Could you check a few things on this model? Use its own coordinates, in mm. A direction names the side the tool comes from. Round coordinates to 2 decimals unless told otherwise and drop trailing zeros. Loops run counter-clockwise (first coordinate to the right, second up) from the corner with the lowest first, then second, coordinate; pieces in that order, holes last.
from build123d import *

# Parameters (mm, degrees)
FILLET1_R          = 2
CHAMFER1_SIZE      = 1.5
CUT_EXTRUDE1_DEPTH = 2
CIRPATTERN1_COUNT  = 8
CUT_EXTRUDE2_DEPTH = 2
CIRPATTERN2_COUNT  = 6


with BuildPart() as part:
    # Sketch2 → Revolve1 (revolve)
    with BuildSketch(Plane(origin=(0, 0, 0), x_dir=(0, 0, -1), z_dir=(1, 0, 0)), mode=Mode.PRIVATE) as revolve1_sk:
        Polygon((0, 3.5), (0, 7.5), (10, 7.5), (10, 8.5), (17, 8.5), (17, 16.166666667), (23, 24.166666667), (23, 41), (21, 41), (21, 43.5), (25, 43.5), (25, 23.5), (19, 15.5), (19, 7), (23, 7), (23, 6), (30, 6), (30, 0), (23, 0), (23, 2.5), (8, 2.5), (8, 3.5), align=None)
    revolve(revolve1_sk.sketch.rotate(Axis((0, 0, 54.509359295), (0, 0, -1)), 90), axis=Axis((0, 0, 54.509359295), (0, 0, -1)))

    # Fillet1
    fillet1_edges = [part.edges().sort_by_distance(p)[0] for p in [
        (-15.5, 0, -19),
        (-23.5, 0, -25),
        (-43.5, 0, -25),
        (-24.166666667, 0, -23),
        (-16.166666667, 0, -17),
    ]]
    fillet(fillet1_edges, radius=FILLET1_R)

    # Chamfer1
    chamfer1_edges = [part.edges().sort_by_distance(p)[0] for p in [
        (-6, 0, -30),
    ]]
    chamfer(chamfer1_edges, length=CHAMFER1_SIZE)

    # Sketch3 → Cut-Extrude1 (cut)
    with BuildSketch(Plane(origin=(0, 0, -25), x_dir=(-1, 0, 0), z_dir=(0, 0, -1))):
        with BuildLine():
            Line((-10.689139417, 31.03211721), (-10.493410806, 30.559586543))
            ThreePointArc((-10.493410806, 30.559586543), (-8.269260882, 28.084064394), (-4.984011152, 27.552851628))
            ThreePointArc((-4.984011152, 27.552851628), (0, 28), (4.984011152, 27.552851628))
            ThreePointArc((4.984011152, 27.552851628), (8.269260882, 28.084064394), (10.493410806, 30.559586543))
            Line((10.493410806, 30.559586543), (10.689139417, 31.03211721))
            ThreePointArc((10.689139417, 31.03211721), (10.46255391, 35.333672006), (6.975673359, 37.862778308))
            ThreePointArc((6.975673359, 37.862778308), (0, 38.5), (-6.975673359, 37.862778308))
            ThreePointArc((-6.975673359, 37.862778308), (-10.46255391, 35.333672006), (-10.689139417, 31.03211721))
        make_face()
    cut_extrude1 = extrude(amount=-CUT_EXTRUDE1_DEPTH, mode=Mode.SUBTRACT)

    # CirPattern1: Cut-Extrude1 ×8 about axis
    cirpattern1_axis = Axis((0, 0, 0), (0, 0, 1))
    for i in range(1, CIRPATTERN1_COUNT):
        add(cut_extrude1.rotate(cirpattern1_axis, i * 360 / CIRPATTERN1_COUNT), mode=Mode.SUBTRACT)

    # Sketch4 → Cut-Extrude2 (cut)
    with BuildSketch(Plane(origin=(0, 0, -19), x_dir=(-1, 0, 0), z_dir=(0, 0, -1))):
        with BuildLine():
            Line((-5.025517215, 11.70445115), (-3.470657901, 9.011355821))
            ThreePointArc((-3.470657901, 9.011355821), (-2.775231815, 8.388165182), (-1.845876826, 8.297152448))
            ThreePointArc((-1.845876826, 8.297152448), (0, 8.5), (1.845876826, 8.297152448))
            ThreePointArc((1.845876826, 8.297152448), (2.775231815, 8.388165182), (3.470657901, 9.011355821))
            Line((3.470657901, 9.011355821), (5.025517215, 11.70445115))
            ThreePointArc((5.025517215, 11.70445115), (5.120456748, 13.008370226), (4.156457468, 13.891503206))
            ThreePointArc((4.156457468, 13.891503206), (0, 14.5), (-4.156457468, 13.891503206))
            ThreePointArc((-4.156457468, 13.891503206), (-5.120456748, 13.008370226), (-5.025517215, 11.70445115))
        make_face()
    cut_extrude2 = extrude(amount=-CUT_EXTRUDE2_DEPTH, mode=Mode.SUBTRACT)

    # CirPattern2: Cut-Extrude2 ×6 about axis
    cirpattern2_axis = Axis((0, 0, 0), (0, 0, 1))
    for i in range(1, CIRPATTERN2_COUNT):
        add(cut_extrude2.rotate(cirpattern2_axis, i * 360 / CIRPATTERN2_COUNT), mode=Mode.SUBTRACT)


solid = part.part
Item 1: If I drill on line 1 along Y through (x, z) = (0, -16.5); line 2 along Y through (x, z) = (13, -21.5); line 3 along Y through (x, z) = (0, -3.5), over which ranges is the centre line in solid material (lowest first)?
Results list:
line 1: y = -8.5 to -2.5, 2.5 to 8.5
line 2: y = -41.51 to -38.88, -17.95 to -13.63, 13.63 to 17.95, 38.88 to 41.51
line 3: y = -7.5 to -3.5, 3.5 to 7.5
Item 2: For faces 3 (the flat face through (-2, 2, -8)), 4 (the flat face through (-3.2, -1.8, 0)), 5 (the cylindrical face through (-17.65, 32.4, -24.01)), which set-ups out of +Z, -Z, +X, -X, +Y, -Y let a thin tool reach every point of the face, with its end or its side?
Results list:
face 3: +Z
face 4: +Z, +X, -X, +Y, -Y
face 5: +Z, -Z
Item 3: If we section it at A-A, the plane y = 0: Count the separate pieces of the cut face and the enclosed holes in it, then the cut area to 3 significant figures.
Results list:
separate pieces: 3
enclosed holes: 0
area: 424 mm2
Item 4: We'd pull the mould along Y, two halves only. Please class faces 1 (the cylindrical face through (-27.154, -27.293, -24.014)), 2 (the flat face through (0, 0, -30)): released by +Y, released by -Y, zero draft, split by the parting line, or undercut.
Results list:
face 1: undercut
face 2: zero draft
Item 5: If we section it at B-B, the plane z = -12.5: Please give me the cut outline in (x, y).
Results list:
outline: circle Ø17 at (0, 0); hole circle Ø5 at (0, 0)
Item 6: Will these pins go through, and if not, where does the flat tip stop? pin 1 (0.6 mm diameter, centred on x = -11, z = -17.5, fed in from +Y); pin 2 (5 mm diameter, centred on x = 19.5, y = 2.5, fed in from +Z); pin 3 (0.6 mm diameter, centred on x = -10.5, z = -17.5, fed in from -Y).
Results list:
pin 1: stops at y = 13.32
pin 2: stops at z = -17.74
pin 3: stops at y = -13.71
